Check sheet for the modelled part. Datum: model origin and axes. Units: mm. Round coordinates to 2 decimals unless told otherwise and drop trailing zeros. Order: outer loops, then holes, each group sorted by start corner. A loop starts at its lowest first (then second) coordinate and runs counter-clockwise, first axis right, second up. Notation, with made-up numbers: (62, 32) -> (77, 32) arc R9 ccw to (77, 46) -> close; hole circle Ø5 at (-6, 68). An arc over 180 degrees is marked (long way). Use CSV: the item, a comma, the result in double quotes.
```python
from build123d import *

# Parameters (mm, degrees)
SKETCH_1_W      = 52
SKETCH_1_H      = 40
SKETCH_1_R      = 13
SKETCH_1_R_2    = 1.744116192
SKETCH_1_R_3    = 2
EXTRUDE_1_DEPTH = 3
FILLET_1_R      = 3


with BuildPart() as part:
    # 草图1 → 凸台-拉伸1 (new body)
    with BuildSketch(Plane.XY):
        Rectangle(SKETCH_1_W, SKETCH_1_H)
        Circle(SKETCH_1_R, mode=Mode.SUBTRACT)
        with Locations((0, 17.5)):
            Circle(SKETCH_1_R_2, mode=Mode.SUBTRACT)
        with Locations((17.5, 0)):
            Circle(SKETCH_1_R_2, mode=Mode.SUBTRACT)
        with Locations((0, -17.5)):
            Circle(SKETCH_1_R_2, mode=Mode.SUBTRACT)
        with Locations((-17.5, 0)):
            Circle(SKETCH_1_R_2, mode=Mode.SUBTRACT)
        with Locations((-23, 15)):
            Circle(SKETCH_1_R_3, mode=Mode.SUBTRACT)
        with Locations(Location((23, 15, 0), (0, 0, 180))):
            Circle(SKETCH_1_R_3, mode=Mode.SUBTRACT)
        with Locations((23, -15)):
            Circle(SKETCH_1_R_3, mode=Mode.SUBTRACT)
        with Locations(Location((-23, -15, 0), (0, 0, 180))):
            Circle(SKETCH_1_R_3, mode=Mode.SUBTRACT)
    extrude(amount=EXTRUDE_1_DEPTH)

    # 圆角1
    fillet_1_edges = [part.edges().sort_by_distance(p)[0] for p in [
        (-26, 20, 1.5),
        (26, 20, 1.5),
        (26, -20, 1.5),
        (-26, -20, 1.5),
    ]]
    fillet(fillet_1_edges, radius=FILLET_1_R)


solid = part.part
```
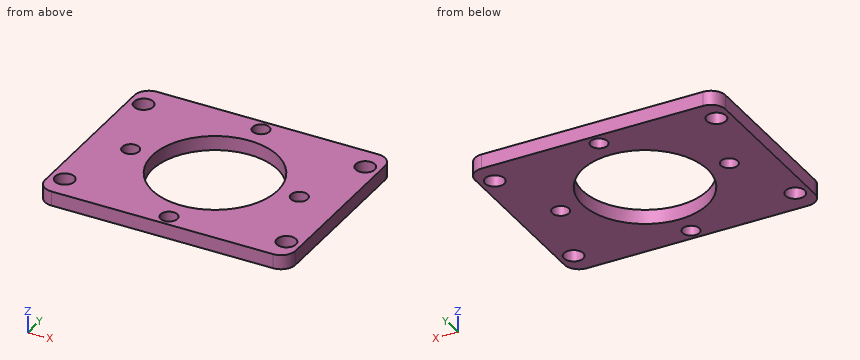
Q1. Go/stop test with a flat-tipped pin: pin 1 (5.5 mm diameter, centred on x = 0, y = 17.5, fed in from +Z). Record where the tip stops, or that it passes through.
Result sheet:
pin 1,"stops at z = 3"
Q2. Sectioned sample at C-C, the plane z = 2.4. State how many separate pieces and enclosed holes the cut face has, then the cut area to 3 significant figures.
Result sheet:
separate pieces,"1"
enclosed holes,"9"
area,"1,450 mm^2"
Q3. Scan lines: L1, parallel to X at y = 14.5, z = 1.95; L2, parallel to X at y = 13.5, z = 2.35; L3, parallel to Y at x = -8, z = 2.7. Record each from-to range of solid material in increasing order.
Result sheet:
L1,"x = -26 to -24.94, -21.06 to 21.06, 24.94 to 26"
L2,"x = -26 to -24.32, -21.68 to 21.68, 24.32 to 26"
L3,"y = -20 to -10.25, 10.25 to 20"
Q4. Sectioned sample at A-A, the plane x = 5. Enter the section's corners in (y, z).
Result sheet:
outline,"(-20, 0) -> (-12, 0) -> (-12, 3) -> (-20, 3) -> close; (12, 0) -> (20, 0) -> (20, 3) -> (12, 3) -> close"
Q5. Sectioned sample at D-D, the plane y = 15. Enter the section's corners in (x, z), then the cut area to 3 significant figures.
Result sheet:
outline,"(-26, 0) -> (-25, 0) -> (-25, 3) -> (-26, 3) -> close; (-21, 0) -> (21, 0) -> (21, 3) -> (-21, 3) -> close; (25, 0) -> (26, 0) -> (26, 3) -> (25, 3) -> close"
area,"132 mm^2"
Q6. Sectioned sample at B-B, the plane y = -12. Enter the section's corners in (x, z).
Result sheet:
outline,"(-26, 0) -> (-5, 0) -> (-5, 3) -> (-26, 3) -> close; (5, 0) -> (26, 0) -> (26, 3) -> (5, 3) -> close"
